The model under review builds one solid part; all positions refer to its coordinate system, in mm. Face numbers are marked on the shaded views. Round coordinates to 2 decimals unless told otherwise and drop trailing zeros. Order: outer loops, then holes, each group sorted by start corner. A loop starts at its lowest first (then second) coordinate and runs counter-clockwise, first axis right, second up. Notation, with made-up numbers: M -4.75,-32 L 5.25,-32 A23 ccw 5.25,-19 Z; hole C 17.25,32.5 d4. An arc over 180 degrees is marked long. Use a Markdown table: item, result. Add a question column.
1. Consider section B-B on x = 0. State the section outline as (y, z) points.
2. Consider section D-D on y = 189.5. State the section outline as (x, z) points, then the cut area to 3 significant figures.
3. To check wall thickness, follow probe 1 along Y at (x, z) = (0, -15.5); probe 2 along X at (y, z) = (183, -15.3); probe 3 along Y at (x, z) = (-7.5, -13.25). State the ranges of each line that lie inside material, in increasing order.
4. Consider section C-C on z = -13.5. State the section outline as (x, y) points.
5. Insertion check: P1, Ø5, axis at x = -9.5, y = 159, coming from the -Z side; P2, Ø4, axis at x = 0, y = 189.5, coming from the +Z side; P3, Ø1.5, axis at x = 9, z = -12.5, coming from the +Y side. Each pin has a flat end and moves straight along its axis. Give the tip position at first contact, or say it passes through.
6. The part is to be moulded in two halves that separate along Y. For the marked faces 1, 2 and 3, say which applies: +Y half, -Y half, draft (parallel to the pull), parting line (faces both ways), or undercut.
7. Consider section A-A on y = 183. State the section outline as (x, z) points.
from build123d import *

# Parameters (mm, degrees)
SKETCH030_W     = 30
SKETCH030_H     = 44
SKETCH030_R     = 2.2
SKETCH030_R_2   = 1.7
PAD016_DEPTH    = 6
CHAMFER007_SIZE = 7
CHAMFER008_SIZE = 0.4


with BuildPart() as part:
    # Sketch030 → Pad016 (new body)
    with BuildSketch(Plane.XY):
        Rectangle(SKETCH030_W, SKETCH030_H)
        with Locations((9.5, 12)):
            Circle(SKETCH030_R, mode=Mode.SUBTRACT)
        with Locations((-9.5, 12)):
            Circle(SKETCH030_R, mode=Mode.SUBTRACT)
        with Locations((-9.5, -12)):
            Circle(SKETCH030_R, mode=Mode.SUBTRACT)
        with Locations((9.5, -12)):
            Circle(SKETCH030_R, mode=Mode.SUBTRACT)
        with Locations((0, 18.5)):
            Circle(SKETCH030_R_2, mode=Mode.SUBTRACT)
        with Locations((0, -18.5)):
            Circle(SKETCH030_R_2, mode=Mode.SUBTRACT)
    extrude(amount=PAD016_DEPTH)

    # Chamfer007
    chamfer007_edges = [part.edges().sort_by_distance(p)[0] for p in [
        (15, 22, 3),
        (-15, 22, 3),
        (-15, -22, 3),
        (15, -22, 3),
    ]]
    chamfer(chamfer007_edges, length=CHAMFER007_SIZE)

    # Chamfer008
    chamfer008_edges = [part.edges().sort_by_distance(p)[0] for p in [
        (-15, 0, 6),
        (-11.5, -18.5, 6),
        (-11.5, 18.5, 6),
        (0, -22, 6),
        (0, 22, 6),
        (11.5, -18.5, 6),
        (11.5, 18.5, 6),
        (15, 0, 6),
        (7.3, 12, 6),
        (-11.7, 12, 6),
        (-11.7, -12, 6),
        (7.3, -12, 6),
        (-1.7, 18.5, 6),
        (-1.7, -18.5, 6),
        (-15, 0, 0),
        (-11.5, -18.5, 0),
        (-11.5, 18.5, 0),
        (0, -22, 0),
        (0, 22, 0),
        (11.5, -18.5, 0),
        (11.5, 18.5, 0),
        (15, 0, 0),
        (7.3, 12, 0),
        (-11.7, 12, 0),
        (-11.7, -12, 0),
        (7.3, -12, 0),
        (-1.7, 18.5, 0),
        (-1.7, -18.5, 0),
    ]]
    chamfer(chamfer008_edges, length=CHAMFER008_SIZE)


with BuildPart() as part_1:
    # Body011 placement: moved
    add(part.part.moved(Location((0, 171, -17.3))))


solid = part_1.part
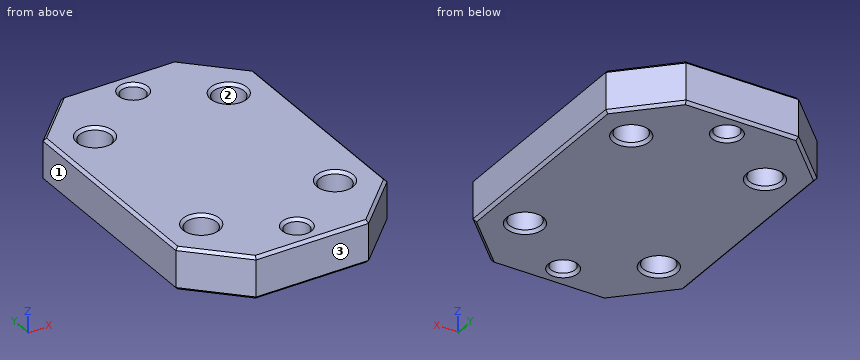
Answer block:
| question | item | result |
|---|---|---|
| 1 | outline | M 149,-16.9 L 149.4,-17.3 L 150.4,-17.3 L 150.8,-16.9 L 150.8,-11.7 L 150.4,-11.3 L 149.4,-11.3 L 149,-11.7 Z; M 154.2,-16.9 L 154.6,-17.3 L 187.4,-17.3 L 187.8,-16.9 L 187.8,-11.7 L 187.4,-11.3 L 154.6,-11.3 L 154.2,-11.7 Z; M 191.2,-16.9 L 191.6,-17.3 L 192.6,-17.3 L 193,-16.9 L 193,-11.7 L 192.6,-11.3 L 191.6,-11.3 L 191.2,-11.7 Z |
| 2 | outline | M -11.5,-16.9 L -10.93,-17.3 L -2.1,-17.3 L -1.7,-16.9 L -1.7,-11.7 L -2.1,-11.3 L -10.93,-11.3 L -11.5,-11.7 Z; M 1.7,-16.9 L 2.1,-17.3 L 10.93,-17.3 L 11.5,-16.9 L 11.5,-11.7 L 10.93,-11.3 L 2.1,-11.3 L 1.7,-11.7 Z |
| 2 | area | 117 mm^2 |
| 3 | probe 1 | 149 to 150.8, 154.2 to 187.8, 191.2 to 193 |
| 3 | probe 2 | -15 to -11.7, -7.3 to 7.3, 11.7 to 15 |
| 3 | probe 3 | 149 to 158.08, 159.92 to 182.08, 183.92 to 193 |
| 4 | outline | M -15,156 L -8,149 L 8,149 L 15,156 L 15,186 L 8,193 L -8,193 L -15,186 Z; hole C -9.5,159 d4.4; hole C -9.5,183 d4.4; hole C 0,152.5 d3.4; hole C 0,189.5 d3.4; hole C 9.5,159 d4.4; hole C 9.5,183 d4.4 |
| 5 | P1 | z = -17.2 |
| 5 | P2 | z = -11.4 |
| 5 | P3 | y = 192.75 |
| 6 | face 1 | draft |
| 6 | face 2 | undercut |
| 6 | face 3 | -Y half |
| 7 | outline | M -15,-16.9 L -14.6,-17.3 L -12.1,-17.3 L -11.7,-16.9 L -11.7,-11.7 L -12.1,-11.3 L -14.6,-11.3 L -15,-11.7 Z; M -7.3,-16.9 L -6.9,-17.3 L 6.9,-17.3 L 7.3,-16.9 L 7.3,-11.7 L 6.9,-11.3 L -6.9,-11.3 L -7.3,-11.7 Z; M 11.7,-16.9 L 12.1,-17.3 L 14.6,-17.3 L 15,-16.9 L 15,-11.7 L 14.6,-11.3 L 12.1,-11.3 L 11.7,-11.7 Z |
